Input: part model. Units: mm. Frame: model coordinates. Face numbers are marked on the shaded views. A direction names the side the tool comes from. Coordinates: 2 decimals unless noted, no trailing zeros. Write each loop counter-clockwise with the first axis right and the second up, starting at its lowest first coordinate (ties: lowest second). Pieces come first, ordered by that corner, then holes. Notation, with made-up numbers: (17, 31) - (26, 31) arc R11 ccw to (26, 37) - close; hole circle Ø2 at (-2.5, -12). An arc over 180 degrees is marked (long way). Use CSV: the item, a comma, the result in double quotes.
```python
from build123d import *

# Parameters (mm, degrees)
BASE_EXTRUDE_DEPTH = 6.35
FILLET1_R          = 6.35
SKETCH2_R          = 2.38125
CUT_EXTRUDE1_DEPTH = 31.986763807


with BuildPart() as part:
    # Sketch1 → Base-Extrude (new, symmetric)
    with BuildSketch(Plane(origin=(0, 0, 0), x_dir=(1, 0, 0), z_dir=(0, 1, 0))):
        with BuildLine():
            Line((-30.1625, 0), (-15.875, 0))
            ThreePointArc((-15.875, 0), (-13.282623356, -0.5532696), (-11.141989448, -2.116666667))
            ThreePointArc((-11.141989448, -2.116666667), (-10.071672494, -2.8983652), (-8.775484171, -3.175))
            Line((-8.775484171, -3.175), (8.775484171, -3.175))
            ThreePointArc((8.775484171, -3.175), (10.071672494, -2.8983652), (11.141989448, -2.116666667))
            ThreePointArc((11.141989448, -2.116666667), (13.282623356, -0.5532696), (15.875, 0))
            Line((15.875, 0), (30.1625, 0))
            Line((30.1625, 0), (30.1625, -3.175))
            Line((30.1625, -3.175), (15.875, -3.175))
            ThreePointArc((15.875, -3.175), (14.578811678, -3.4516348), (13.508494724, -4.233333333))
            ThreePointArc((13.508494724, -4.233333333), (11.367860816, -5.7967304), (8.775484171, -6.35))
            Line((8.775484171, -6.35), (-8.775484171, -6.35))
            ThreePointArc((-8.775484171, -6.35), (-11.367860816, -5.7967304), (-13.508494724, -4.233333333))
            ThreePointArc((-13.508494724, -4.233333333), (-14.578811678, -3.4516348), (-15.875, -3.175))
            Line((-15.875, -3.175), (-30.1625, -3.175))
            Line((-30.1625, -3.175), (-30.1625, 0))
        make_face()
    extrude(amount=BASE_EXTRUDE_DEPTH, both=True)

    # Fillet1
    fillet1_edges = [part.edges().sort_by_distance(p)[0] for p in [
        (30.1625, -6.35, 1.5875),
        (-30.1625, -6.35, 1.5875),
        (30.1625, 6.35, 1.5875),
        (-30.1625, 6.35, 1.5875),
    ]]
    fillet(fillet1_edges, radius=FILLET1_R - 0.0001)  # a hair under: the kernel refuses the full size

    # Sketch2 → Cut-Extrude1 (cut, through all)
    with BuildSketch(Plane.XY.offset(3.175)):
        with Locations((23.8125, 0)):
            Circle(SKETCH2_R)
        with Locations((-23.8125, 0)):
            Circle(SKETCH2_R)
    extrude(amount=-CUT_EXTRUDE1_DEPTH, mode=Mode.SUBTRACT)


solid = part.part
```
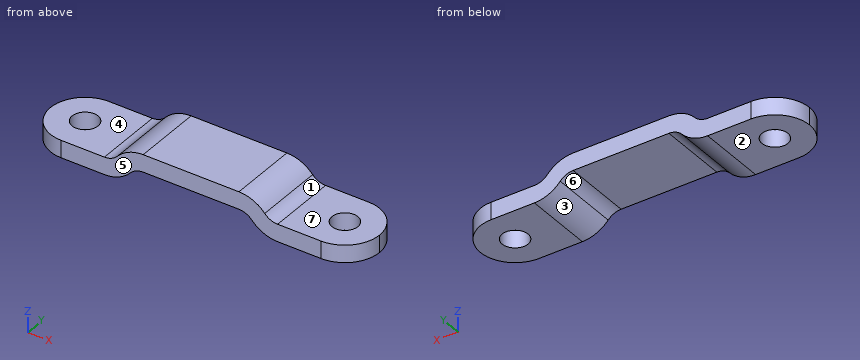
(1) Cut plane D-D on x = -1. Return loops of the section in (y, z) (3 decimals).
Check values:
outline,"(-6.35, 3.175) - (6.35, 3.175) - (6.35, 6.35) - (-6.35, 6.35) - close"
(2) Reachability of the marked faces 4, 5, 6 and 7 from +Z, -Z, +X, -X, +Y, -Y: full face, straight path, thin tool, end or side. Return the list, or none.
Check values:
face 4,"+Z, -X, +Y, -Y"
face 5,"+Z, -Z, +X, -X, -Y"
face 6,"-Z, +Y, -Y"
face 7,"+Z, +X, +Y, -Y"
(3) Cut plane A-A on z = 1.5. State how many separate pieces and enclosed holes the cut face has, and give its area (3 significant figures).
Check values:
separate pieces,"2"
enclosed holes,"2"
area,"397 mm^2"
(4) Draft query along X for the marked faces 1, 2 and 3. Return one class per face: pulls with the +X half, pulls with the -X half, needs draft (parallel to the pull), parting line crosses it, or undercut.
Check values:
face 1,"pulls with the +X half"
face 2,"needs draft"
face 3,"undercut"
(5) Cut plane C-C on x = -22.5. Return loops of the section in (y, z) (3 decimals).
Check values:
outline,"(-6.35, 0) - (-1.987, 0) - (-1.987, 3.175) - (-6.35, 3.175) - close; (1.987, 0) - (6.35, 0) - (6.35, 3.175) - (1.987, 3.175) - close"
(6) Ray query, probe 1 along X at (y, z) = (-1.25, 2); probe 2 along Z at (x, y) = (-6, 3.75) (3 decimals); probe 3 along X at (y, z) = (2.5, 2.5). Return the intervals inside material, ascending. Write a range as from..to.
Check values:
probe 1,"-30.04..-25.84, -21.79..-11.25, 11.25..21.79, 25.84..30.04"
probe 2,"3.175..6.35"
probe 3,"-29.65..-10.73, 10.73..29.65"
(7) Pin query (flat end, axial travel): pin 1 Ø4 at (x, y) = (23, 0) entering from +Z (3 decimals); pin 2 Ø3 at (y, z) = (-4, 4) entering from -X; pin 3 Ø3 at (x, z) = (1, 1.5) entering from +Y; pin 4 Ø4 at (x, y) = (-2, -1) entering from -Z (3 decimals). Return the tip coordinate at first contact, or that it passes through.
Check values:
pin 1,"z = 3.175"
pin 2,"x = -29.54"
pin 3,"through"
pin 4,"z = 3.175"
